from build123d import *

# Parameters (mm, degrees)
BOSS_EXTRUDE2_DEPTH = 88.9
SKETCH8_W           = 5.93725
SKETCH8_H           = 12.7
CUT_EXTRUDE3_DEPTH  = 92.025212307
SKETCH10_W          = 5.93725
SKETCH10_H          = 12.7
CUT_EXTRUDE4_DEPTH  = 92.025212307


with BuildPart() as part:
    # Sketch4 → Boss-Extrude2 (new body)
    with BuildSketch(Plane(origin=(0, 0, 0), x_dir=(1, 0, 0), z_dir=(0, 1, 0))):
        with BuildLine():
            Line((0, 0), (0, -19.05))
            Line((0, -19.05), (1.016, -19.05))
            Line((1.016, -19.05), (1.016, 0))
            ThreePointArc((1.016, 0), (3.365064987, 0.274963066), (1.143, -0.535060511))
            Line((1.143, -0.535060511), (1.143, -1.933363843))
            ThreePointArc((1.143, -1.933363843), (4.106126962, 1.122980938), (0, 0))
        make_face()
    extrude(amount=BOSS_EXTRUDE2_DEPTH)

    # Sketch8 → Cut-Extrude3 (cut, through all)
    with BuildSketch(Plane(origin=(0, 0, 0), x_dir=(0, 0, -1), z_dir=(1, 0, 0))):
        with Locations((0, 6.35)):
            Rectangle(SKETCH8_W, SKETCH8_H)
        with Locations((0, 31.75)):
            Rectangle(SKETCH8_W, SKETCH8_H)
        with Locations((0, 57.15)):
            Rectangle(SKETCH8_W, SKETCH8_H)
        with Locations((0, 82.55)):
            Rectangle(SKETCH8_W, SKETCH8_H)
    extrude(amount=CUT_EXTRUDE3_DEPTH, mode=Mode.SUBTRACT)

    # Sketch10 → Cut-Extrude4 (cut, through all)
    with BuildSketch(Plane(origin=(0, 0, 0), x_dir=(0, 0, -1), z_dir=(1, 0, 0))):
        with Locations((0, 44.45)):
            Rectangle(SKETCH10_W, SKETCH10_H)
    extrude(amount=CUT_EXTRUDE4_DEPTH, mode=Mode.SUBTRACT)


solid = part.part
Design review of the part built by this model. Coordinates are the model's own, in mm. A direction names the side the tool comes from. Give positions to 0.01 mm unless a question says otherwise; leave off trailing zeros. Loops run counter-clockwise (first coordinate to the right, second up) from the corner with the lowest first, then second, coordinate; pieces in that order, holes last. Notation, with made-up numbers: (-1.5, 7.25) - (46.5, 7.25) arc R29 cw to (46.5, 41.25) - close; hole circle Ø4 at (-25.5, 78). An arc over 180 degrees is marked (long way). Use CSV: the item, a comma, the result in double quotes. Start each with the question number.
1. Add section A-A (y = 78). State the section outline as (x, z) points.
2. Insertion check: P1, Ø1, axis at x = 3, y = 74.5, coming from the +Z side; P2, Ø1, axis at y = 70, z = 11, coming from the +X side; P3, Ø0.5, axis at x = 0.5, y = 7.5, coming from the -Z side; P4, Ø1.4, axis at x = 2.21, z = 0, coming from the +Y side. Each pin has a flat end and moves straight along its axis. Give the tip position at first contact, or say it passes through.
3. Machinability: for faces 4 (the cylindrical face through (3.353, 69.761, -0.322)), 5 (the flat face through (1, 12.7, -1)), 6 (the flat face through (1, 25.4, -1)), 7 (the flat face through (1, 76.2, -1)), which of the approach directions +Z, -Z, +X, -X, +Y, -Y give a long, thin tool a straight path to every point of the face, cutting with its end or side? Answer none if there is none.
4. Draft analysis for pull direction Z (two halves, no side actions). For faces 1 (the cylindrical face through (4.146, 18.961, -1.053)), 2 (the flat face through (1, 63.5, -1)), 3 (the cylindrical face through (3.353, 18.961, -0.322)), state which applies: released by +Z, released by -Z, zero draft, split by the parting line, or undercut.
5. Wall thickness on L1, parallel to Y at x = 2.5, z = 1.5; L2, parallel to X at y = 18, z = 18.25; L3, parallel to X at y = 67, z = -0.75: over which ranges is each line inside the solid? List them lowest first.
6. Add section B-B (z = 17.5). State the section outline as (x, y) points.
Results found:
1,outline,"(0, 2.97) - (1.02, 2.97) - (1.02, 19.05) - (0, 19.05) - close"
2,P1,"stops at z = 2.19"
2,P2,"stops at x = 1.02"
2,P3,"stops at z = 2.97"
2,P4,"passes through"
3,face 4,"+Y, -Y"
3,face 5,"-Z, +X, -X, -Y"
3,face 6,"-Z, +X, -X"
3,face 7,"-Z, +X, -X, +Y"
4,face 1,"split by the parting line"
4,face 2,"zero draft"
4,face 3,"undercut"
5,L1,"y = 12.7 to 25.4, 63.5 to 76.2"
5,L2,"x = 0 to 1.02"
5,L3,"x = 0.13 to 1.28, 3.13 to 4.28"
6,outline,"(0, 0) - (1.02, 0) - (1.02, 88.9) - (0, 88.9) - close"
